from build123d import *

# Parameters (mm, degrees)
F0_R     = 8.65
F0_R_2   = 6.65
F1_DEPTH = 11
F3_R     = 13.6
F3_R_2   = 11.6
F4_DEPTH = 7
F8_DEPTH = 0.5
F10_R    = 5


with BuildPart() as f1:
    # F0 (on Top) → F1 (new body)
    with BuildSketch(Plane.XY):
        Circle(F0_R)
        Circle(F0_R_2, mode=Mode.SUBTRACT)
    extrude(amount=F1_DEPTH)


with BuildPart() as f4:
    # F3 (on offset) → F4 (new body)
    with BuildSketch(Plane.XY.offset(17)):
        Circle(F3_R)
        Circle(F3_R_2, mode=Mode.SUBTRACT)
    extrude(amount=F4_DEPTH)


with BuildPart() as f6:
    # F5 (on Front) → F6 (revolve)
    with BuildSketch(Plane.XZ):
        Polygon((11.6, 17), (6.65, 11), (8.65, 11), (13.6, 17), align=None)
    revolve(axis=Axis((0, 0, 14), (0, 0, 1)))


with BuildPart() as f8:
    # F7 (on offset) → F8 (new body)
    with BuildSketch(Plane.XY.offset(17)):
        with BuildLine():
            Line((-5, -11.018621), (-5, 11.018621))
            ThreePointArc((-5, 11.018621), (-6.02744, 10.4919), (-7, 9.86965))
            Line((-7, 9.86965), (-7, -9.86965))
            ThreePointArc((-7, -9.86965), (-6.02744, -10.4919), (-5, -11.018621))
        make_face()
        with BuildLine():
            Line((1, -12.058607), (1, 12.058607))
            ThreePointArc((1, 12.058607), (0.500428, 12.089647), (0, 12.1))
            Line((0, 12.1), (0, 0))
            Line((0, 0), (0, -12.1))
            ThreePointArc((0, -12.1), (0.500428, -12.089647), (1, -12.058607))
        make_face()
        with BuildLine():
            Line((0, 0), (0, 12.1))
            ThreePointArc((0, 12.1), (-0.500428, 12.089647), (-1, 12.058607))
            Line((-1, 12.058607), (-1, -12.058607))
            ThreePointArc((-1, -12.058607), (-0.500428, -12.089647), (0, -12.1))
            Line((0, -12.1), (0, 0))
        make_face()
        with BuildLine():
            Line((7, -9.86965), (7, 9.86965))
            ThreePointArc((7, 9.86965), (6.02744, 10.4919), (5, 11.018621))
            Line((5, 11.018621), (5, -11.018621))
            ThreePointArc((5, -11.018621), (6.02744, -10.4919), (7, -9.86965))
        make_face()
    extrude(amount=F8_DEPTH)


with BuildPart() as f1_1:
    add(f1.part)

    # F9: union F6, F4, F8
    add(f6.part)
    add(f4.part)
    add(f8.part)

    # F10
    f10_edges = [f1_1.edges().sort_by_distance(p)[0] for p in [
        (-8.65, 0, 11),
        (-13.6, 0, 17),
    ]]
    fillet(f10_edges, radius=F10_R)


solid = f1_1.part
Read the model definition and answer for the solid it produces. Units are mm, in the model's axes. A direction names the side the tool comes from. Coordinates: 2 decimals unless noted, no trailing zeros. Order: outer loops, then holes, each group sorted by start corner. A loop starts at its lowest first (then second) coordinate and runs counter-clockwise, first axis right, second up. Notation, with made-up numbers: M 21.5,21.5 L 36.5,21.5 A11 ccw 36.5,26.5 Z; hole C -36,54 d4. An arc over 180 degrees is marked long. Put each result on its own line as item: value. Start each with the question number.
Item 1: Section B-B, the plane z = 6 is taken. Determine the outline of the cut face in (x, y).
Item 2: Consider probe 1 along X at (y, z) = (0, 20); probe 2 along Y at (x, z) = (0, 6.25). Determine where each line is inside the solid, lowest interval first. Write a range as [from, to].
Item 3: The mould has two halves that part along X. Classify faces 4 (the face through (-6, 0, 17)), 5 (the face through (-8.64, 0.38, 4.54)), 6 (the face through (2.5, -6.4, 0)), 7 (the face through (3.07, -5.9, 5.42)): +X half, -X half, draft (parallel to the pull), parting line (faces both ways), or undercut.
Item 4: Given pin 1 Ø2 at (x, y) = (4, 5) entering from -Z; pin 2 Ø3 at (x, z) = (5, 11.5) entering from -Y; pin 3 Ø0.6 at (y, z) = (-2, 17.5) entering from +X; pin 4 Ø1.6 at (x, y) = (-6, -5) entering from +Z, each flat-ended and moving along its own axis, determine where each tip first touches the part or whether it passes through.
Item 5: Section A-A, the plane y = 0 is taken. Count the separate pieces of the cut face and the enclosed holes in it, plus the area to 3 significant figures.
Item 6: For faces 1 (the face through (-6, 0, 17.5)), 2 (the face through (6, 0, 17)), 3 (the face through (11.02, 4.09, 24)), determine the directions among +Z, -Z, +X, -X, +Y, -Y from which every point of the face is accessible in a straight line to the end or side of a thin tool.
Computed:
1. outline: C 0,0 d17.3; hole C 0,0 d13.3
2. probe 1: x = [-13.6, -11.6], [11.6, 13.6]
2. probe 2: y = [-8.65, -6.65], [6.65, 8.65]
3. face 4: undercut
3. face 5: parting line
3. face 6: draft
3. face 7: undercut
4. pin 1: stops at z = 0
4. pin 2: stops at y = -9.2
4. pin 3: stops at x = 13.36
4. pin 4: stops at z = 17.5
5. separate pieces: 5
5. enclosed holes: 0
5. area: 99.0 mm2
6. face 1: +Z
6. face 2: none
6. face 3: +Z, +X, -X, +Y, -Y
